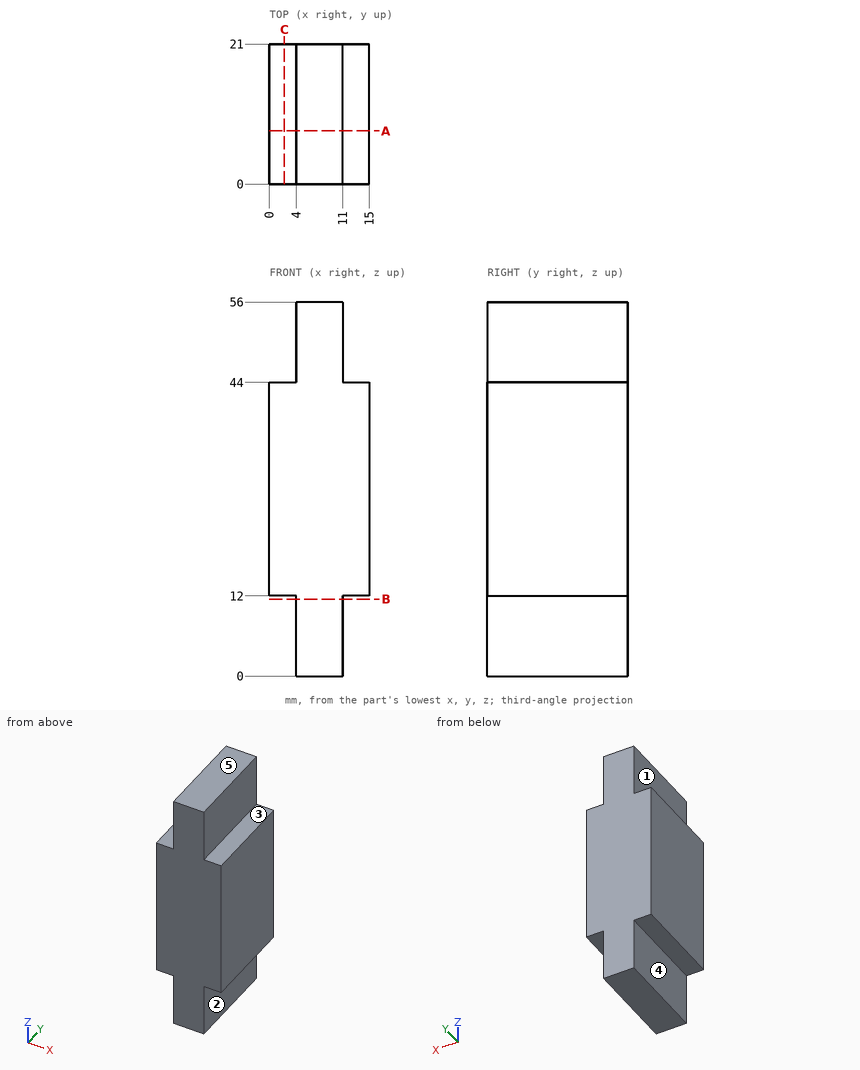
Here's the drawing with two shaded views (mm, measured from the low corner). I have some questions. A direction names the side the tool comes from. Give positions to 0.01 mm unless a question says otherwise; leave off trailing zeros. Write each loop counter-clockwise with the first axis right and the second up, starting at its lowest first coordinate (ties: lowest second). Pieces come first, ordered by that corner, then holes. Notation, with made-up numbers: (12, 5.5) -> (70, 5.5) arc R28 ccw to (70, 29.5) -> close; hole circle Ø3 at (80, 6). An arc over 180 degrees is marked (long way). Use one line per item in the form item = value. Start each with the question number.
1. Imagine slicing it at C-C on x = 2.25. List the corners of the cut face in (y, z) for me.
2. Imagine slicing it at B-B on z = 11.5. List the corners of the cut face in (x, y) for me.
3. Will these pins go through, and if not, where does the flat tip stop? pin 1 Ø3 at (y, z) = (15, 50.5) entering from +X; pin 2 Ø2 at (x, y) = (13, 9.5) entering from +Z; pin 3 Ø3.5 at (y, z) = (10.5, 7) entering from -X.
4. Imagine slicing it at A-A on y = 8. List the corners of the cut face in (x, z) for me, plus the area to 3 significant figures.
5. On a 3-axis mill with a long thin cutter (end or side, diameter ignored), from which of +Z, -Z, +X, -X, +Y, -Y can I reach the whole of each face in a straight line? I mean the marked faces 1, 2, 3, 4 and 5. Say none if no direction works.
6. If I drill on L1, parallel to X at y = 19.75, z = 8.5; L2, parallel to Z at x = 11.5, y = 1.25, over which ranges is the centre line in solid material (lowest first)?
Entries:
q1.outline = (0, 12) -> (21, 12) -> (21, 44) -> (0, 44) -> close
q2.outline = (4, 0) -> (11, 0) -> (11, 21) -> (4, 21) -> close
q3.pin_1 = 11
q3.pin_2 = 44
q3.pin_3 = 4
q4.outline = (0, 12) -> (4, 12) -> (4, 0) -> (11, 0) -> (11, 12) -> (15, 12) -> (15, 44) -> (11, 44) -> (11, 56) -> (4, 56) -> (4, 44) -> (0, 44) -> close
q4.area = 648 mm²
q5.face_1 = +Z, -X, +Y, -Y
q5.face_2 = -Z, +X, +Y, -Y
q5.face_3 = +Z, +X, +Y, -Y
q5.face_4 = -Z, -X, +Y, -Y
q5.face_5 = +Z, +X, -X, +Y, -Y
q6.L1 = 4 to 11
q6.L2 = 12 to 44
